Part model, mm, in its own coordinate system. A direction names the side the tool comes from. Round coordinates to 2 decimals unless told otherwise and drop trailing zeros. Write each loop counter-clockwise with the first axis right and the second up, starting at its lowest first coordinate (ties: lowest second). Pieces come first, ordered by that corner, then holes. Notation, with made-up numbers: M 12.5,84.5 L 52.5,84.5 A31 ccw 52.5,122.5 Z; hole C -4.75,20.25 d9. An arc over 180 degrees is marked long. Use one line per item in the form item = value. Start each with the question number.
Item 1: Flat gauge pins, fed straight in: pin 1 Ø24 at (x, y) = (12.5, -75.5) entering from +Z; pin 2 Ø22 at (x, z) = (21.5, 67) entering from +Y. Where does each tip first touch, or does it go through?
Item 2: Cut at C-C, the plane x = -37.5. Give the cut face in (y, z).
Item 3: Mould opens along Y. For faces 3 (the face through (-1, 0, 1)), 4 (the face through (-1, -115, 1)), 5 (the face through (-1, -24, 75)) say: +Y half, -Y half, draft (parallel to the pull), parting line (faces both ways), or undercut.
Item 4: Probe L1, parallel to X at y = -79.5, z = -16; L2, parallel to Y at x = -8.5, z = -52; L3, parallel to Z at x = -51, y = -115.5. List the from-to ranges inside material, lowest first.
Item 5: Which spindle directions (+Z, -Z, +X, -X, +Y, -Y) get a long thin tool onto all of the face, cutting with end or side? Do faces 1 (the face through (-1, -74, -55)), 2 (the face through (80, -74, -1)). Say none if no direction does.
Item 6: Cut at A-A, the plane z = 12. Give the cut face in (x, y), then the cut area to 3 significant figures.
Item 7: Cut at B-B, the plane y = -65.5. Give the cut face in (x, z).
from build123d import *

# Parameters (mm, degrees)
F0_W     = 160
F0_H     = 150
F1_DEPTH = 150
F2_W     = 120
F2_H     = 100
F3_DEPTH = 20
F4_W     = 100
F4_H     = 80
F5_DEPTH = 110


with BuildPart() as f1:
    # F0 (on Front) → F1 (new body)
    with BuildSketch(Plane.XZ):
        Rectangle(F0_W, F0_H)
    extrude(amount=F1_DEPTH)

    # F2 (on face) → F3 (cut)
    with BuildSketch(Plane.XY.offset(75)):
        with Locations((0, -75)):
            Rectangle(F2_W, F2_H)
    extrude(amount=-F3_DEPTH, mode=Mode.SUBTRACT)

    # F4 (on face) → F5 (cut)
    with BuildSketch(Plane.XY.offset(55)):
        with Locations((0, -75)):
            Rectangle(F4_W, F4_H)
    extrude(amount=-F5_DEPTH, mode=Mode.SUBTRACT)


solid = f1.part
Model answer:
q1.pin_1 = -55
q1.pin_2 = 0
q2.outline = M -150,-75 L 0,-75 L 0,75 L -25,75 L -25,55 L -35,55 L -35,-55 L -115,-55 L -115,55 L -125,55 L -125,75 L -150,75 Z
q3.face_3 = +Y half
q3.face_4 = undercut
q3.face_5 = draft
q4.L1 = -80 to -50, 50 to 80
q4.L2 = -150 to -115, -35 to 0
q4.L3 = -75 to 55
q5.face_1 = +Z
q5.face_2 = +Z, -Z, +X, +Y, -Y
q6.outline = M -80,-150 L 80,-150 L 80,0 L -80,0 Z; hole M -50,-115 L 50,-115 L 50,-35 L -50,-35 Z
q6.area = 16,000 mm²
q7.outline = M -80,-75 L 80,-75 L 80,75 L 60,75 L 60,55 L 50,55 L 50,-55 L -50,-55 L -50,55 L -60,55 L -60,75 L -80,75 Z
